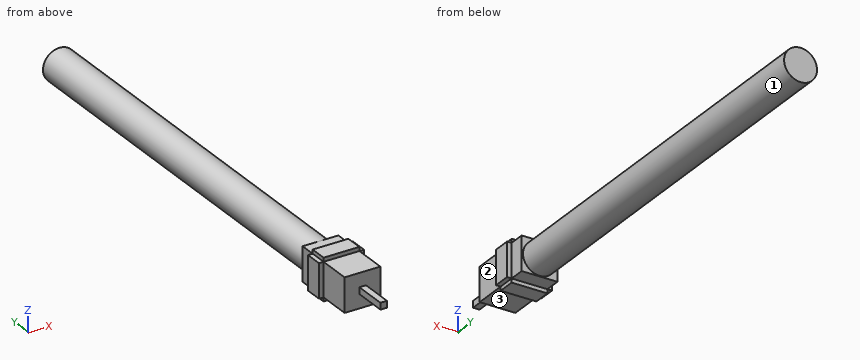
from build123d import *

# Parameters (mm, degrees)
F0_R      = 6.35
F1_DEPTH  = 78.994
F3_W      = 13.791928
F3_H      = 13.131412
F4_DEPTH  = 25.4
F5_W      = 6.633806
F5_H      = 13.131412
F6_DEPTH  = 1.778
F7_W      = 13.791928
F7_H      = 6.633806
F8_DEPTH  = 1.524
F11_W     = 2.54
F11_H     = 2.54
F12_DEPTH = 12.7


with BuildPart() as f1:
    # F0 (on Front) → F1 (new body)
    with BuildSketch(Plane.XZ):
        Circle(F0_R)
    extrude(amount=F1_DEPTH)

    # F2: F1 across plane


with BuildPart() as f1_1:
    add(f1.part)
    add(f1.part.mirror(Plane.XZ))

    # F3 (on face) → F4 (join)
    with BuildSketch(Plane.XZ.offset(78.994)):
        Rectangle(F3_W, F3_H)
    extrude(amount=F4_DEPTH)

    # F5 (on face) → F6 (join)
    with BuildSketch(Plane(origin=(-6.895964, 0, 0), x_dir=(0, -1, 0), z_dir=(-1, 0, 0))):
        with Locations((88.377097, 0)):
            Rectangle(F5_W, F5_H)
    extrude(amount=F6_DEPTH)

    # F7 (on face) → F8 (join)
    with BuildSketch(Plane(origin=(0, 0, -6.565706), x_dir=(1, 0, 0), z_dir=(0, 0, -1))):
        with Locations((0, 88.377097)):
            Rectangle(F7_W, F7_H)
    extrude(amount=F8_DEPTH)

    # F9: F1 across plane


with BuildPart() as f1_2:
    add(f1_1.part)
    add(f1_1.part.mirror(Plane.YZ))

    # F10: F1 across plane


with BuildPart() as f1_3:
    add(f1_2.part)
    add(f1_2.part.mirror(Plane.XY))

    # F11 (on face) → F12 (join)
    with BuildSketch(Plane.XZ.offset(104.394)):
        with Locations((0.104479, 0.000465)):
            Rectangle(F11_W, F11_H)
    extrude(amount=F12_DEPTH)


solid = f1_3.part
Geometry check sheet. Reference: the model listing, model coordinates, mm. Face numbers are marked on the shaded views. A direction names the side the tool comes from. Coordinates: 2 decimals unless noted, no trailing zeros. Loops run counter-clockwise (first coordinate to the right, second up) from the corner with the lowest first, then second, coordinate; pieces in that order, holes last. Notation, with made-up numbers: (60, -27) - (110, -27) arc R24 cw to (110, -14) - close; hole circle Ø8 at (20, 26). An arc over 180 degrees is marked (long way). Use one line per item in the form item = value. Start each with the question number.
Item 1: Section check B-B, the plane y = -19.5. Enter the section's corners in (x, z).
Item 2: Thickness scan on probe 1 along Y at (x, z) = (-1.5, -1); probe 2 along Y at (x, z) = (-3.5, -6.25); probe 3 along X at (y, z) = (-93.5, 4.75). Record the ranges inside material, lowest first.
Item 3: Section check A-A, the plane x = -4.75. Enter the section's corners in (y, z), and give its area (3 significant figures).
Item 4: Gauge pin test, flat ends, axial feed: pin 1 (5 mm diameter, centred on y = -82, z = 0.5, fed in from +X); pin 2 (1 mm diameter, centred on x = -6, y = 40.5, fed in from -Z); pin 3 (1.4 mm diameter, centred on x = -7.5, z = -0.5, fed in from -Y). Record the tip position at first contact, or that the pin passes through.
Item 5: Tool access check on the marked faces 1, 2 and 3. Record the directions out of +Z, -Z, +X, -X, +Y, -Y that give a thin tool (end or side, any length) a straight path to the whole face; none if there is none.
Item 6: Section check C-C, the plane x = 3.5. Enter the section's corners in (y, z), and give its area (3 significant figures).
Computed:
q1.outline = circle Ø12.7 at (0, 0)
q2.probe_1 = -104.39 to 78.99
q2.probe_2 = -104.39 to -78.99
q2.probe_3 = -6.9 to 6.9
q3.outline = (-104.39, -6.57) - (-91.69, -6.57) - (-91.69, -8.09) - (-85.06, -8.09) - (-85.06, -6.57) - (-78.99, -6.57) - (-78.99, -4.21) - (78.99, -4.21) - (78.99, 4.21) - (-78.99, 4.21) - (-78.99, 6.57) - (-85.06, 6.57) - (-85.06, 8.09) - (-91.69, 8.09) - (-91.69, 6.57) - (-104.39, 6.57) - close
q3.area = 1,690 mm2
q4.pin_1 = 6.9
q4.pin_2 = -3.17
q4.pin_3 = -104.39
q5.face_1 = +Y
q5.face_2 = +Z, -Z, +X, -Y
q5.face_3 = -Z, +X, -X, -Y
q6.outline = (-104.39, -6.57) - (-91.69, -6.57) - (-91.69, -8.09) - (-85.06, -8.09) - (-85.06, -6.57) - (-78.99, -6.57) - (-78.99, -5.3) - (78.99, -5.3) - (78.99, 5.3) - (-78.99, 5.3) - (-78.99, 6.57) - (-85.06, 6.57) - (-85.06, 8.09) - (-91.69, 8.09) - (-91.69, 6.57) - (-104.39, 6.57) - close
q6.area = 2,030 mm2
